Can you work these out from the drawing? Everything is in mm from the part's minimum corner. Coordinates: 2 decimals unless noted, no trailing zeros. Loops run counter-clockwise (first coordinate to the right, second up) from the corner with the lowest first, then second, coordinate; pieces in that order, holes last. Notation, with made-up numbers: (-26, 88) -> (-15, 88) arc R24 ccw to (-15, 106) -> close; hole circle Ø4 at (3.25, 81.25). An arc over 180 degrees is marked (long way). One line per question, with ' | ' between items.
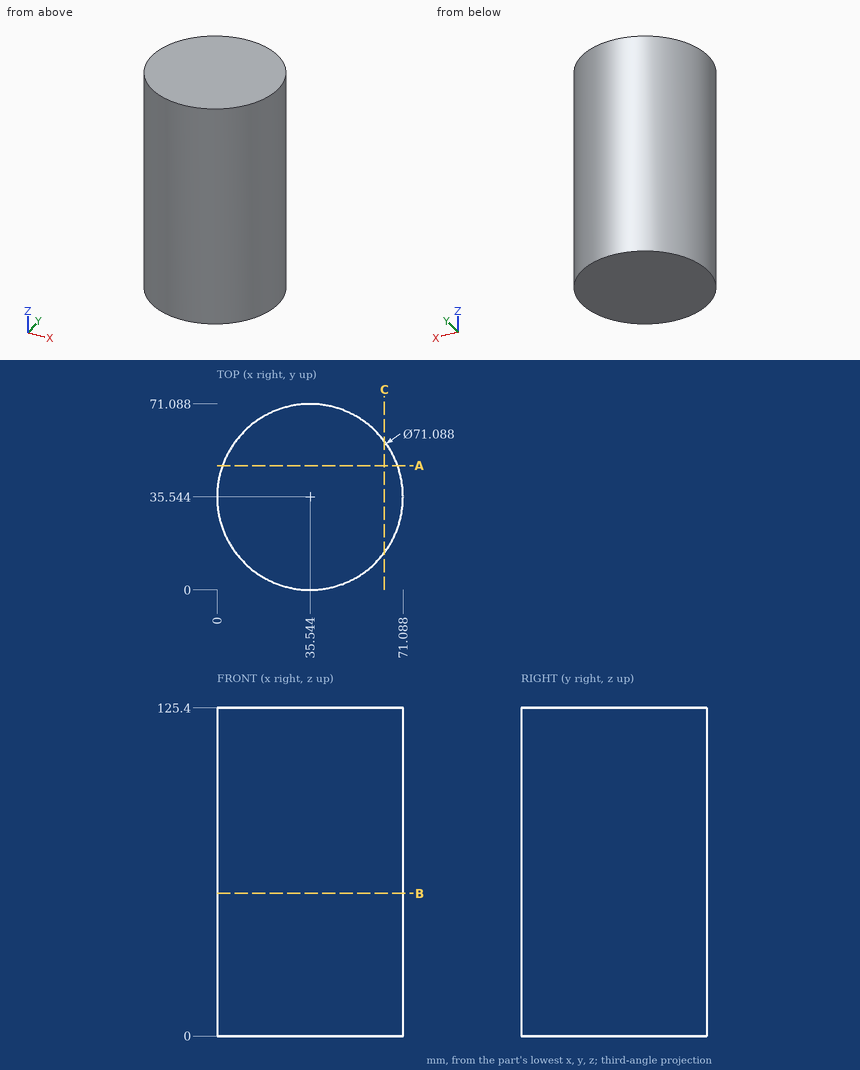
Q1. Imagine slicing it at C-C on x = 64. Write out the boundary of the cut face in (y, z) (1 decimal), plus the area to 3 significant figures.
Values follow:
outline: (14.2, 0) -> (56.8, 0) -> (56.8, 125.4) -> (14.2, 125.4) -> close | area: 5,340 mm2
Q2. Imagine slicing it at A-A on y = 47.5. Write out the boundary of the cut face in (x, z).
Values follow:
outline: (2.07, 0) -> (69.02, 0) -> (69.02, 125.4) -> (2.07, 125.4) -> close
Q3. Imagine slicing it at B-B on z = 54.5. Write out the boundary of the cut face in (x, y).
Values follow:
outline: circle Ø71.09 at (35.54, 35.54)
Q4. Please list where these lines run through material, in increasing order: L1, parallel to X at y = 53.5, z = 13; L2, parallel to Y at x = 17, z = 119; L3, parallel to X at y = 66.5, z = 8 (1 decimal). Write a range as [from, to].
Values follow:
L1: x = [4.87, 66.22] | L2: y = [5.22, 65.87] | L3: x = [18.1, 53]
Q5. For pin 1 (2 mm diameter, centred on y = 54, z = 105, fed in from -X); pin 2 (10 mm diameter, centred on y = 26, z = 93, fed in from +X); pin 3 (6 mm diameter, centred on x = 8, z = 35, fed in from +Y), each with a flat end and sliding along its axis, tell me the tip position at first contact or that it passes through.
Values follow:
pin 1: stops at x = 4.58 | pin 2: stops at x = 70.8 | pin 3: stops at y = 61.25
